Design review of the part built by this model. Coordinates are the model's own, in mm. A direction names the side the tool comes from. Coordinates: 2 decimals unless noted, no trailing zeros. Write each loop counter-clockwise with the first axis right and the second up, starting at its lowest first coordinate (ties: lowest second). Pieces come first, ordered by that corner, then holes.
Q1. Take a section at B-B, the plane z = 25. Write out the cut boundary in (x, y), plus the area to 3 significant figures.
Q2. The part is to be moulded in two halves that separate along Y. For faces 1 (the flat face through (-43, 6.5, 7)), 2 (the flat face through (33, 16, -41.599)), 3 (the cylindrical face through (-46.5, 4.07, -44.2)), say which applies: released by +Y, released by -Y, zero draft, split by the parting line, or undercut.
Q3. Take a section at A-A, the plane y = 16.5. Write out the cut boundary in (x, z).
Q4. Take a section at C-C, the plane x = 1. Write out the cut boundary in (y, z).
Q5. For pin 1 Ø0.8 at (y, z) = (16, -41) entering from -X; pin 2 Ø6.5 at (x, y) = (-35.5, 17.5) entering from -Z; pin 3 Ø1.9 at (x, z) = (34, 41) entering from -Y, all flat-tipped, find the tip position at first contact; note any pin that passes through.
Q6. Take a section at D-D, the plane x = -37.65. Write out the cut boundary in (y, z), plus the area to 3 significant figures.
Q7. For faces 4 (the flat face through (-45, 4, -40.5)), 5 (the cylindrical face through (45.29, 2.77, 32)), 6 (the flat face through (-32, 3.5, -41)), 7 (the cylindrical face through (32, 2.77, 45.21)), 8 (the flat face through (21, 5, 41)), list the 3-axis set-ups (+Z, -Z, +X, -X, +Y, -Y) from which the entire face can be reached by the end or side of a thin tool; tool diameter is ignored.
Q8. For L1, parallel to X at y = 5.75, z = 23; L2, parallel to Z at x = 41, y = 6, list the stretches that pass through material, from the lowest coordinate up.
from build123d import *

# Parameters (mm, degrees)
SKETCH1_W                                            = 96
SKETCH1_H                                            = 96
SKETCH1_W_2                                          = 80
SKETCH1_H_2                                          = 80
BOSS_EXTRUDE1_DEPTH                                  = 8
F_3_0_3_DIAMETER_HOLE3_D                             = 3
F_3_0_3_DIAMETER_HOLE3_DEPTH                         = 7.5
SKETCH27_W                                           = 82
SKETCH27_H                                           = 82
CUT_EXTRUDE2_DEPTH                                   = 10
F_3_0_3_DIAMETER_HOLE1_D                             = 3
F_3_4_3_4_DIAMETER_HOLE1_D                           = 3.4
SKETCH38_W                                           = 85
SKETCH38_H                                           = 85
CUT_EXTRUDE4_DEPTH                                   = 10
F_3_0_3_DIAMETER_HOLE7_D                             = 3
SKETCH44_W                                           = 4
SKETCH44_H                                           = 4
BOSS_EXTRUDE2_DEPTH                                  = 8
SKETCH45_W                                           = 4
SKETCH45_H                                           = 3.5
BOSS_EXTRUDE3_DEPTH                                  = 8
SKETCH49_W                                           = 96
SKETCH49_H                                           = 1.5
CUT_EXTRUDE5_DEPTH                                   = 146
TAP_DRILL_FOR_M4_TAP1_D                              = 4
SKETCH53_W                                           = 4
SKETCH53_H                                           = 6.5
BOSS_EXTRUDE5_DEPTH                                  = 78
SKETCH54_W                                           = 16
SKETCH54_H                                           = 1.5
SKETCH54_W_2                                         = 16.883483494
BOSS_EXTRUDE6_DEPTH                                  = 18.5
FILLET1_R                                            = 0.5
SKETCH57_W                                           = 4
SKETCH57_H                                           = 6.5
CUT_EXTRUDE6_DEPTH                                   = 7.5
SKETCH58_W                                           = 4
SKETCH58_H                                           = 6.5
BOSS_EXTRUDE7_DEPTH                                  = 81
FILLET2_R                                            = 0.5
SKETCH61_W                                           = 32
SKETCH61_H                                           = 85
CUT_EXTRUDE7_DEPTH                                   = 81
CSK_FOR_M2_5_COUNTERSUNK_FLAT_HEAD_SCREW_D           = 2.5
CSK_FOR_M2_5_COUNTERSUNK_FLAT_HEAD_SCREW_DEPTH       = 7.901
CSK_FOR_M2_5_COUNTERSUNK_FLAT_HEAD_SCREW_CSINK_D     = 5
CSK_FOR_M2_5_COUNTERSUNK_FLAT_HEAD_SCREW_CSINK_ANGLE = 90
CSK_FOR_M2_5_COUNTERSUNK_FLAT_HEAD_S_2_D             = 2.5
CSK_FOR_M2_5_COUNTERSUNK_FLAT_HEAD_S_2_DEPTH         = 7.901
CSK_FOR_M2_5_COUNTERSUNK_FLAT_HEAD_S_2_CSINK_D       = 5
CSK_FOR_M2_5_COUNTERSUNK_FLAT_HEAD_S_2_CSINK_ANGLE   = 90
SKETCH66_W                                           = 85
SKETCH66_H                                           = 80.198
CUT_EXTRUDE8_DEPTH                                   = 10
SKETCH67_W                                           = 85
SKETCH67_H                                           = 85
CUT_EXTRUDE9_DEPTH                                   = 3.5
SKETCH68_W                                           = 42
SKETCH68_H                                           = 85
CUT_EXTRUDE10_DEPTH                                  = 56


with BuildPart() as part:
    # Sketch1 → Boss-Extrude1 (new body)
    with BuildSketch(Plane(origin=(0, 0, 0), x_dir=(1, 0, 0), z_dir=(0, 1, 0))):
        Rectangle(SKETCH1_W, SKETCH1_H)
        Rectangle(SKETCH1_W_2, SKETCH1_H_2, mode=Mode.SUBTRACT)
    extrude(amount=BOSS_EXTRUDE1_DEPTH)

    # Ø3.0 (3) Diameter Hole3
    with Locations(Plane(origin=(0, 0, -48), x_dir=(-1, 0, 0), z_dir=(0, 0, -1))):
        with Locations((45, 4)):
            Hole(F_3_0_3_DIAMETER_HOLE3_D / 2, depth=F_3_0_3_DIAMETER_HOLE3_DEPTH)

    # Sketch27 → Cut-Extrude2 (cut)
    with BuildSketch(Plane(origin=(0, 8, 0), x_dir=(1, 0, 0), z_dir=(0, 1, 0))):
        Rectangle(SKETCH27_W, SKETCH27_H)
    extrude(amount=-CUT_EXTRUDE2_DEPTH, mode=Mode.SUBTRACT)

    # Ø3.0 (3) Diameter Hole1 (through all)
    with Locations(Plane.XY.offset(48)):
        with Locations((-30.5, 2.7), (30.5, 2.7)):
            Hole(F_3_0_3_DIAMETER_HOLE1_D / 2)

    # Ø3.4 (3.4) Diameter Hole1 (through all)
    with Locations(Plane(origin=(0, 0, 0), x_dir=(-1, 0, 0), z_dir=(0, -1, 0))):
        with Locations((-23, 45.5), (23, 45.5), (45.5, 23), (45.5, -25), (23, -45.5), (-23, -45.5), (-45.5, -25), (-45.5, 25)):
            Hole(F_3_4_3_4_DIAMETER_HOLE1_D / 2)

    # Sketch38 → Cut-Extrude4 (cut)
    with BuildSketch(Plane(origin=(0, 8, 0), x_dir=(1, 0, 0), z_dir=(0, 1, 0))):
        Rectangle(SKETCH38_W, SKETCH38_H)
    extrude(amount=-CUT_EXTRUDE4_DEPTH, mode=Mode.SUBTRACT)

    # Ø3.0 (3) Diameter Hole7 (through all)
    with Locations(Plane.ZY.offset(48)):
        with Locations((-30.5, 2.7), (30.5, 2.7)):
            Hole(F_3_0_3_DIAMETER_HOLE7_D / 2)

    # Sketch44 → Boss-Extrude2 (add)
    with BuildSketch(Plane.XZ):
        with Locations((40.5, -40.5)):
            Rectangle(SKETCH44_W, SKETCH44_H)
        with Locations((-40.5, -40.5)):
            Rectangle(SKETCH44_W, SKETCH44_H)
        with Locations((-40.5, 40.5)):
            Rectangle(SKETCH44_W, SKETCH44_H)
        with Locations((40.5, 40.5)):
            Rectangle(SKETCH44_W, SKETCH44_H)
    extrude(amount=-BOSS_EXTRUDE2_DEPTH)

    # Sketch45 → Boss-Extrude3 (add)
    with BuildSketch(Plane(origin=(0, 8, 0), x_dir=(1, 0, 0), z_dir=(0, 1, 0))):
        with Locations((-40.5, 36.75)):
            Rectangle(SKETCH45_W, SKETCH45_H)
    extrude(amount=-BOSS_EXTRUDE3_DEPTH)

    # Sketch49 → Cut-Extrude5 (cut)
    with BuildSketch(Plane(origin=(48, 0, 0), x_dir=(0, 0, -1), z_dir=(1, 0, 0))):
        with Locations((0, 7.25)):
            Rectangle(SKETCH49_W, SKETCH49_H)
    extrude(amount=-CUT_EXTRUDE5_DEPTH, mode=Mode.SUBTRACT)

    # Tap Drill for M4 Tap1 (through all)
    with Locations(Plane(origin=(0, 6.5, 0), x_dir=(1, 0, 0), z_dir=(0, 1, 0))):
        with Locations((44.6, -44.6), (-44.6, -44.6), (44.6, 44.6)):
            Hole(TAP_DRILL_FOR_M4_TAP1_D / 2)

    # Sketch53 → Boss-Extrude5 (add)
    with BuildSketch(Plane(origin=(-38.5, 0, 0), x_dir=(0, 0, -1), z_dir=(1, 0, 0))):
        with Locations((-40.5, 3.25)):
            Rectangle(SKETCH53_W, SKETCH53_H)
    extrude(amount=BOSS_EXTRUDE5_DEPTH)

    # Sketch54 → Boss-Extrude6 (add)
    with BuildSketch(Plane(origin=(0, 6.5, 0), x_dir=(1, 0, 0), z_dir=(0, 1, 0))):
        with Locations((33, -40.849)):
            Rectangle(SKETCH54_W, SKETCH54_H)
        with Locations((-33.441741747, -40.849)):
            Rectangle(SKETCH54_W_2, SKETCH54_H)
        with Locations((33.441741747, 40.849)):
            Rectangle(SKETCH54_W_2, SKETCH54_H)
    extrude(amount=BOSS_EXTRUDE6_DEPTH)

    # Fillet1
    fillet1_edges = [part.edges().sort_by_distance(p)[0] for p in [
        (41, 6.5, 40.849),
        (25, 6.5, 40.849),
        (33, 6.5, 41.599),
        (-41.883483494, 6.5, 40.849),
        (-33.441741747, 6.5, 41.599),
        (-25, 6.5, 40.849),
    ]]
    fillet(fillet1_edges, radius=FILLET1_R)

    # Sketch57 → Cut-Extrude6 (cut)
    with BuildSketch(Plane.XY.offset(-35)):
        with Locations((-40.5, 3.25)):
            Rectangle(SKETCH57_W, SKETCH57_H)
    extrude(amount=-CUT_EXTRUDE6_DEPTH, mode=Mode.SUBTRACT)

    # Sketch58 → Boss-Extrude7 (add)
    with BuildSketch(Plane.ZY.offset(-38.5)):
        with Locations((-40.5, 3.25)):
            Rectangle(SKETCH58_W, SKETCH58_H)
    extrude(amount=BOSS_EXTRUDE7_DEPTH)

    # Fillet2
    fillet2_edges = [part.edges().sort_by_distance(p)[0] for p in [
        (41.883483494, 6.5, -40.849),
        (33.441741747, 6.5, -41.599),
        (25, 6.5, -40.849),
    ]]
    fillet(fillet2_edges, radius=FILLET2_R)

    # Sketch61 → Cut-Extrude7 (cut)
    with BuildSketch(Plane(origin=(0, 6.5, 0), x_dir=(1, 0, 0), z_dir=(0, 1, 0))):
        Rectangle(SKETCH61_W, SKETCH61_H)
    extrude(amount=-CUT_EXTRUDE7_DEPTH, mode=Mode.SUBTRACT)

    # CSK for M2.5 Countersunk Flat Head Screw
    with Locations(Plane.XY.offset(-40.099)):
        with Locations((28.15, 21.825324496), (37.65, 21.825324496)):
            CounterSinkHole(CSK_FOR_M2_5_COUNTERSUNK_FLAT_HEAD_SCREW_D / 2, CSK_FOR_M2_5_COUNTERSUNK_FLAT_HEAD_SCREW_CSINK_D / 2, depth=CSK_FOR_M2_5_COUNTERSUNK_FLAT_HEAD_SCREW_DEPTH, counter_sink_angle=CSK_FOR_M2_5_COUNTERSUNK_FLAT_HEAD_SCREW_CSINK_ANGLE)

    # CSK for M2.5 Countersunk Flat Head S 2
    with Locations(Plane(origin=(0, 0, 40.099), x_dir=(-1, 0, 0), z_dir=(0, 0, -1))):
        with Locations((-28.15, 21.825324496), (-37.65, 21.825324496), (28.15, 21.825324496), (37.65, 21.825324496)):
            CounterSinkHole(CSK_FOR_M2_5_COUNTERSUNK_FLAT_HEAD_S_2_D / 2, CSK_FOR_M2_5_COUNTERSUNK_FLAT_HEAD_S_2_CSINK_D / 2, depth=CSK_FOR_M2_5_COUNTERSUNK_FLAT_HEAD_S_2_DEPTH, counter_sink_angle=CSK_FOR_M2_5_COUNTERSUNK_FLAT_HEAD_S_2_CSINK_ANGLE)

    # Sketch66 → Cut-Extrude8 (cut)
    with BuildSketch(Plane(origin=(0, 6.5, 0), x_dir=(1, 0, 0), z_dir=(0, 1, 0))):
        Rectangle(SKETCH66_W, SKETCH66_H)
    extrude(amount=-CUT_EXTRUDE8_DEPTH, mode=Mode.SUBTRACT)

    # Sketch67 → Cut-Extrude9 (cut)
    with BuildSketch(Plane.XZ):
        Rectangle(SKETCH67_W, SKETCH67_H)
    extrude(amount=-CUT_EXTRUDE9_DEPTH, mode=Mode.SUBTRACT)

    # Sketch68 → Cut-Extrude10 (cut)
    with BuildSketch(Plane(origin=(0, 6.5, 0), x_dir=(1, 0, 0), z_dir=(0, 1, 0))):
        Rectangle(SKETCH68_W, SKETCH68_H)
    extrude(amount=-CUT_EXTRUDE10_DEPTH, mode=Mode.SUBTRACT)


solid = part.part
Responses:
1. outline: (-48, 0) - (-47.2, 0) - (-47.2, 6.5) - (-48, 6.5) - close; (-43.8, 0) - (-42.5, 0) - (-42.5, 6.5) - (-43.8, 6.5) - close; (42.5, 0) - (43.8, 0) - (43.8, 6.5) - (42.5, 6.5) - close; (47.2, 0) - (48, 0) - (48, 6.5) - (47.2, 6.5) - close
1. area: 27.3 mm2
2. face 1: released by +Y
2. face 2: zero draft
2. face 3: undercut
3. outline: (-41.88, 40.1) - (-25, 40.1) - (-25, 41.6) - (-41.88, 41.6) - close; (25, -41.6) - (41.88, -41.6) - (41.88, -40.1) - (25, -40.1) - close; (25, 40.1) - (41, 40.1) - (41, 41.6) - (25, 41.6) - close
4. outline: (0, -48) - (6.5, -48) - (6.5, -42.5) - (0, -42.5) - close; (0, 42.5) - (6.5, 42.5) - (6.5, 48) - (0, 48) - close
5. pin 1: stops at x = 25
5. pin 2: stops at z = 40.1
5. pin 3: stops at y = 3.5
6. outline: (0, -48) - (6.5, -48) - (6.5, -40.1) - (3.5, -40.1) - (3.5, -42.5) - (0, -42.5) - close; (0, 42.5) - (3.5, 42.5) - (3.5, 40.1) - (19.33, 40.1) - (20.58, 41.35) - (20.58, 41.6) - (7, 41.6) arc R0.5 cw to (6.5, 42.1) - (6.5, 48) - (0, 48) - close; (23.08, 41.35) - (24.33, 40.1) - (25, 40.1) - (25, 41.6) - (23.08, 41.6) - close
6. area: 108 mm2
7. face 4: -Z
7. face 5: +X, -X
7. face 6: -Y
7. face 7: +Z
7. face 8: +Y, -Y
8. L1: x = -48 to -42.5, 42.5 to 48
8. L2: z = -48 to -40.1, 40.1 to 48
